Source: CAD feature listing. Evaluate the final solid. Frame: model axes, mm. Face numbers are marked on the shaded views. A direction names the side the tool comes from. Round coordinates to 2 decimals unless told otherwise and drop trailing zeros. Loops run counter-clockwise (first coordinate to the right, second up) from the corner with the lowest first, then second, coordinate; pieces in that order, holes last. Notation, with made-up numbers: M 37.25,2 L 56.25,2 A30 cw 56.25,35 Z; hole C -37.5,79 d4. An arc over 180 degrees is marked long. One line per item, written item: value.
from build123d import *

# Parameters (mm, degrees)
SKETCH1_W           = 22.3
SKETCH1_H           = 12
BOSS_EXTRUDE1_DEPTH = 22.3
SKETCH2_W           = 12
SKETCH2_H           = 2.4
BOSS_EXTRUDE2_DEPTH = 4.5
EXTRUDE_1_DEPTH     = 4.3
SKETCH_1_R          = 0.75
CUT_EXTRUDE_1_DEPTH = 10
SKETCH_2_R          = 2.25
EXTRUDE_2_DEPTH     = 4.2


with BuildPart() as part:
    # Sketch1 → Boss-Extrude1 (new body)
    with BuildSketch(Plane(origin=(0, 0, 0), x_dir=(1, 0, 0), z_dir=(0, 1, 0))):
        Rectangle(SKETCH1_W, SKETCH1_H)
    extrude(amount=BOSS_EXTRUDE1_DEPTH)

    # Sketch2 → Boss-Extrude2 (add)
    with BuildSketch(Plane.ZY.offset(11.15)):
        with Locations((0, 17)):
            Rectangle(SKETCH2_W, SKETCH2_H)
    boss_extrude2 = extrude(amount=BOSS_EXTRUDE2_DEPTH)

    # 镜向1: Boss-Extrude2 across plane
    add(boss_extrude2.mirror(Plane(origin=(0, 0, 0), x_dir=(0, 0, 1), z_dir=(1, 0, 0))))

    # Sketch5 → 凸台-拉伸1 (add)
    with BuildSketch(Plane(origin=(0, 22.3, 0), x_dir=(1, 0, 0), z_dir=(0, 1, 0))):
        with BuildLine():
            Line((0.693260261, 2.906739739), (-0.188814246, 2.906739739))
            ThreePointArc((-0.188814246, 2.906739739), (-10.9, 0), (-0.188814246, -2.906739739))
            Line((-0.188814246, -2.906739739), (0.693260261, -2.906739739))
            ThreePointArc((0.693260261, -2.906739739), (3.6, 0), (0.693260261, 2.906739739))
        make_face()
    extrude(amount=EXTRUDE_1_DEPTH)

    # 草图1 → 切除-拉伸1 (cut)
    with BuildSketch(Plane(origin=(0, 18.2, 0), x_dir=(1, 0, 0), z_dir=(0, 1, 0))):
        with Locations(Location((-13.68, 0, 0), (0, 0, 270))):
            Circle(SKETCH_1_R)
        with Locations(Location((13.68, 0, 0), (0, 0, 270))):
            Circle(SKETCH_1_R)
    extrude(amount=-CUT_EXTRUDE_1_DEPTH, mode=Mode.SUBTRACT)

    # 草图2 → 凸台-拉伸2 (add)
    with BuildSketch(Plane(origin=(0, 26.6, 0), x_dir=(1, 0, 0), z_dir=(0, 1, 0))):
        with Locations(Location((-5.15, 0, 0), (0, 0, 270))):
            Circle(SKETCH_2_R)
    extrude(amount=EXTRUDE_2_DEPTH)


solid = part.part
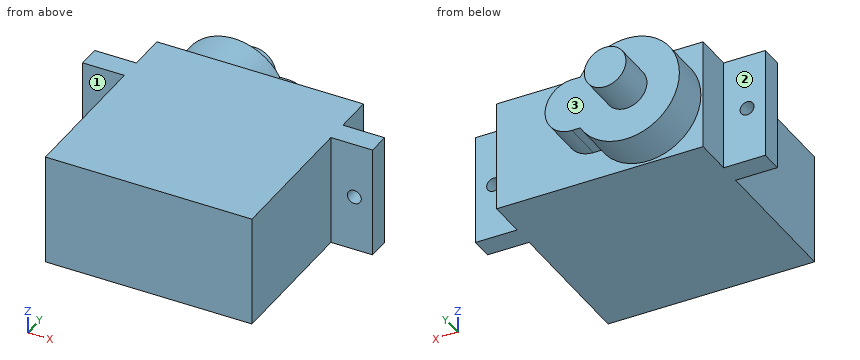
1. Section query D-D (z = 1.75). Return the cut outline in (x, y).
Report:
outline: M -15.65,15.8 L -11.15,15.8 L -11.15,0 L 11.15,0 L 11.15,15.8 L 15.65,15.8 L 15.65,18.2 L 11.15,18.2 L 11.15,22.3 L 3.01,22.3 L 3.01,26.6 L -3.74,26.6 L -3.74,30.8 L -6.56,30.8 L -6.56,26.6 L -10.63,26.6 L -10.63,22.3 L -11.15,22.3 L -11.15,18.2 L -15.65,18.2 Z
2. Ray query, line 1 (X direction, y = 16.65, z = 0); line 2 (X direction, y = 16.5, z = 0.25); line 3 (Y direction, x = -10, z = -1.25). Return the intervals inside material, ascending. Write a range as [from, to].
Report:
line 1: x = [-15.65, -14.43], [-12.93, 12.93], [14.43, 15.65]
line 2: x = [-15.65, -14.39], [-12.97, 12.97], [14.39, 15.65]
line 3: y = [0, 26.6]
3. Section query B-B (x = -13.68). Return the cut outline in (y, z).
Report:
outline: M 15.8,-6 L 18.2,-6 L 18.2,-0.75 L 15.8,-0.75 Z; M 15.8,0.75 L 18.2,0.75 L 18.2,6 L 15.8,6 Z
4. Section query A-A (z = 0). Return the cut outline in (x, y).
Report:
outline: M -15.65,15.8 L -14.43,15.8 L -14.43,18.2 L -15.65,18.2 Z; M -12.93,15.8 L -11.15,15.8 L -11.15,0 L 11.15,0 L 11.15,15.8 L 12.93,15.8 L 12.93,18.2 L 11.15,18.2 L 11.15,22.3 L 3.6,22.3 L 3.6,26.6 L -2.9,26.6 L -2.9,30.8 L -7.4,30.8 L -7.4,26.6 L -10.9,26.6 L -10.9,22.3 L -11.15,22.3 L -11.15,18.2 L -12.93,18.2 Z; M 14.43,15.8 L 15.65,15.8 L 15.65,18.2 L 14.43,18.2 Z
5. Pin query (flat end, axial travel): pin 1 (1.7 mm diameter, centred on x = -13.68, z = 0, fed in from -Y); pin 2 (8 mm diameter, centred on x = 4.5, y = 26.5, fed in from -Z); pin 3 (1.3 mm diameter, centred on x = 13.5, z = -0.5, fed in from +Y). Return the tip coordinate at first contact, or that it passes through.
Report:
pin 1: stops at y = 15.8
pin 2: stops at z = -2.91
pin 3: stops at y = 18.2
6. Section query C-C (x = -5.15). Return the cut outline in (y, z).
Report:
outline: M 0,-6 L 22.3,-6 L 22.3,-5.75 L 26.6,-5.75 L 26.6,-2.25 L 30.8,-2.25 L 30.8,2.25 L 26.6,2.25 L 26.6,5.75 L 22.3,5.75 L 22.3,6 L 0,6 Z
7. Reachability of the marked faces 1, 2 and 3 from +Z, -Z, +X, -X, +Y, -Y: full face, straight path, thin tool, end or side. Return the list, or none.
Report:
face 1: +Z, -Z, -X, -Y
face 2: +Z, -Z, -X, +Y
face 3: +Y
